from build123d import *

# Parameters (mm, degrees)
SKETCH1_W           = 150
SKETCH1_H           = 80
BOSS_EXTRUDE1_DEPTH = 15
SKETCH2_R           = 35.508350292
CUT_EXTRUDE1_DEPTH  = 31
FILLET1_R           = 10


with BuildPart() as part:
    # Sketch1 → Boss-Extrude1 (new body, symmetric)
    with BuildSketch(Plane(origin=(0, 0, 0), x_dir=(1, 0, 0), z_dir=(0, 1, 0))):
        Rectangle(SKETCH1_W, SKETCH1_H)
    extrude(amount=BOSS_EXTRUDE1_DEPTH, both=True)

    # Sketch2 → Cut-Extrude1 (cut, through all)
    with BuildSketch(Plane(origin=(0, 15, 0), x_dir=(1, 0, 0), z_dir=(0, 1, 0))):
        Circle(SKETCH2_R)
    extrude(amount=-CUT_EXTRUDE1_DEPTH, mode=Mode.SUBTRACT)

    # Fillet1
    fillet1_edges = [part.edges().sort_by_distance(p)[0] for p in [
        (75, 0, 40),
        (75, 0, -40),
    ]]
    fillet(fillet1_edges, radius=FILLET1_R)


solid = part.part
Input: part model. Units: mm. Frame: model coordinates. Give positions to 0.01 mm unless a question says otherwise; leave off trailing zeros. Write each loop counter-clockwise with the first axis right and the second up, starting at its lowest first coordinate (ties: lowest second). Pieces come first, ordered by that corner, then holes. Notation, with made-up numbers: M -8.75,0.25 L 19.25,0.25 A26 ccw 19.25,25.25 Z; hole C 50.5,-12.75 d8. An arc over 180 degrees is marked long. Use one line per item in the form item = value.
1. Ray query, L1, parallel to Z at x = 0, y = 5.25; L2, parallel to X at y = -8.75, z = 0; L3, parallel to Z at x = 25, y = 8. Return the intervals inside material, ascending.
Outcome:
L1 = -40 to -35.51, 35.51 to 40
L2 = -75 to -35.51, 35.51 to 75
L3 = -40 to -25.22, 25.22 to 40
2. Cut plane A-A on x = 0. Return loops of the section in (y, z).
Outcome:
outline = M -15,-40 L 15,-40 L 15,-35.51 L -15,-35.51 Z; M -15,35.51 L 15,35.51 L 15,40 L -15,40 Z
3. Cut plane B-B on y = -8. Return loops of the section in (x, z).
Outcome:
outline = M -75,-40 L 65,-40 A10 ccw 75,-30 L 75,30 A10 ccw 65,40 L -75,40 Z; hole C 0,0 d71.02
4. Mould query, pull axis X, two halves, no side actions, for faces 1 (the face through (-6, 0, -40)), 2 (the face through (71.99, 0.21, 37.15)), 3 (the face through (-7.698, 0.21, 34.664)). Classes: released by +X, released by -X, zero draft, split by the parting line, or undercut.
Outcome:
face_1 = zero draft
face_2 = released by +X
face_3 = undercut
5. Cut plane C-C on z = 0. Return loops of the section in (x, y), and give its area (3 significant figures).
Outcome:
outline = M -75,-15 L -35.51,-15 L -35.51,15 L -75,15 Z; M 35.51,-15 L 75,-15 L 75,15 L 35.51,15 Z
area = 2,370 mm²
